Source: three-view drawing plus pictorial views. Frame: mm from the lowest corner of the part. A direction names the side the tool comes from. Give positions to 0.01 mm unless a question says otherwise; leave off trailing zeros. Loops run counter-clockwise (first coordinate to the right, second up) from the corner with the lowest first, then second, coordinate; pieces in that order, holes last. Notation, with made-up numbers: (-36.75, -16.5) -> (-20.75, -16.5) arc R16 cw to (-20.75, -1.5) -> close; hole circle Ø7 at (-32, -31). An arc over 180 degrees is marked (long way). Answer as a JSON object with one key per item and string values. Group by question number.
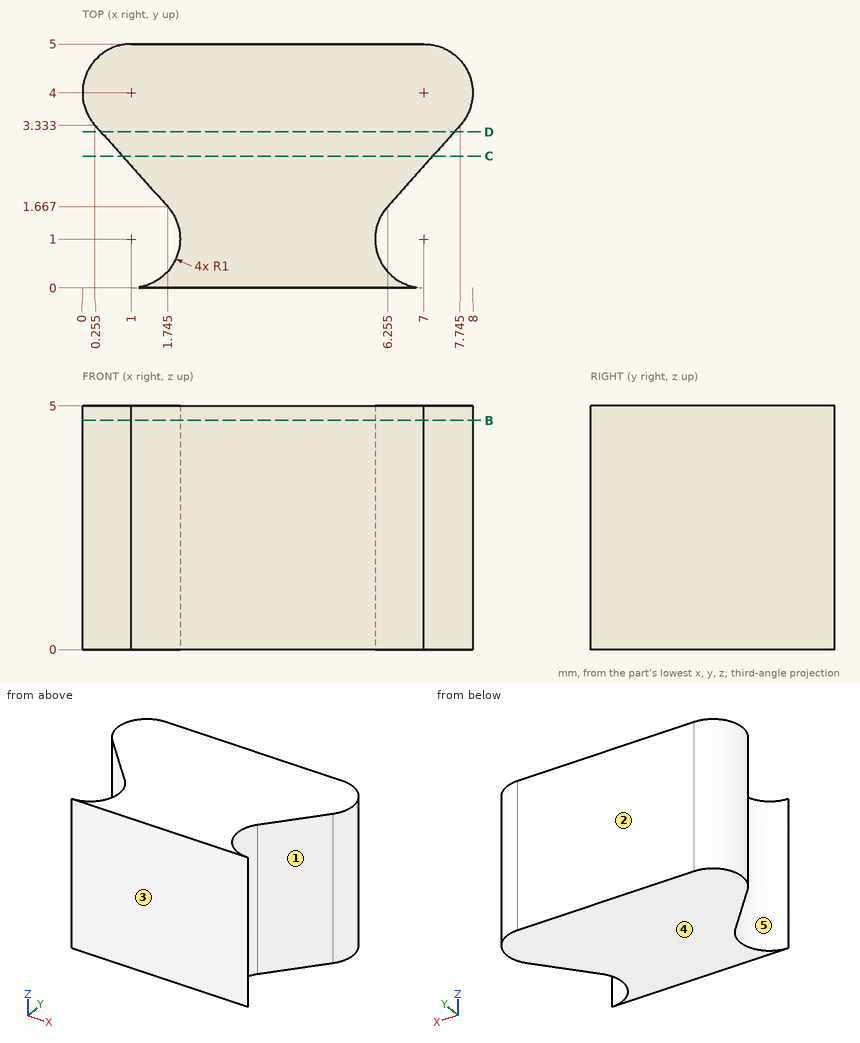
Q1. Section D-D on y = 3.2. Return the cut outline in (x, z).
Q2. Section B-B on z = 4.7. Return the cut outline in (x, y) (1 decimal), then the cut area to 3 significant figures.
Q3. Ray query, probe 1 along X at (y, z) = (1.15, 4.7); probe 2 along X at (y, z) = (4.4, 2.3); probe 3 along Y at (x, z) = (0.5, 1.9) (1 decimal). Return the intervals inside material, ascending.
Q4. Set-up query: the marked faces 1 and 2. Return all of +Z, -Z, +X, -X, +Y, -Y with unobstructed straight access to the full face (end or side cutting, diameter ignored); none if empty.
Q5. Pin query (flat end, axial travel): pin 1 Ø2 at (y, z) = (2.5, 3.5) entering from -X. Return the tip coordinate at first contact, or that it passes through.
Q6. Section C-C on y = 2.7. Return the cut outline in (x, z).
Q7. Pull-direction query (Y, two-part tool) for the marked faces 3, 4 and 5; classes: +Y half, -Y half, draft (parallel to the pull), parting line (faces both ways), or undercut.
Numbers:
{
 "1": {"outline": "(0.37, 0) -> (7.63, 0) -> (7.63, 5) -> (0.37, 5) -> close"},
 "2": {"outline": "(0.3, 3.3) -> (1.7, 1.7) arc R1 cw to (1, 0) -> (7, 0) arc R1 cw to (6.3, 1.7) -> (7.7, 3.3) arc R1 ccw to (7, 5) -> (1, 5) arc R1 ccw to start", "area": "30.0 mm²"},
 "3": {"probe 1": "x = 1.99 to 6.01", "probe 2": "x = 0.08 to 7.92", "probe 3": "y = 3.1 to 4.9"},
 "4": {"face 1": "+Z, -Z, +X", "face 2": "+Z, -Z, +X, -X, +Y"},
 "5": {"pin 1": "stops at x = 0.13"},
 "6": {"outline": "(0.82, 0) -> (7.18, 0) -> (7.18, 5) -> (0.82, 5) -> close"},
 "7": {"face 3": "-Y half", "face 4": "draft", "face 5": "undercut"}
}
